from build123d import *

# Parameters (mm, degrees)
CYLINDER003_R     = 1.25
CYLINDER003_DEPTH = 9
CYLINDER002_R     = 1.25
CYLINDER002_DEPTH = 9
BOX008_W          = 5
BOX008_H          = 25
BOX008_DEPTH      = 10
BOX009_W          = 5
BOX009_H          = 5
BOX009_DEPTH      = 2
BOX005_W          = 20
BOX005_H          = 10
BOX005_DEPTH      = 10
CYLINDER_R        = 6.25
CYLINDER_DEPTH    = 5
CYLINDER001_R     = 7.25
CYLINDER001_DEPTH = 5
BOX004_W          = 6.5
BOX004_H          = 7
BOX004_DEPTH      = 10
BOX002_W          = 13.5
BOX002_H          = 10
BOX002_DEPTH      = 12
BOX003_W          = 13
BOX003_H          = 13
BOX003_DEPTH      = 12
BOX_W             = 17
BOX_H             = 23
BOX_DEPTH         = 12
BOX001_W          = 19
BOX001_H          = 25
BOX001_DEPTH      = 10
BOX007_W          = 13
BOX007_H          = 10
BOX007_DEPTH      = 10
BOX006_W          = 15
BOX006_H          = 10
BOX006_DEPTH      = 10
BOX010_W          = 1
BOX010_H          = 10
BOX010_DEPTH      = 1.6


with BuildPart() as cylinder003:
    # Cylinder003 → Cylinder003 (new body)
    with BuildSketch(Plane(origin=(-2, 20, 1), x_dir=(1, 0, 0), z_dir=(0, 0, 1))):
        Circle(CYLINDER003_R)
    extrude(amount=CYLINDER003_DEPTH)


with BuildPart() as cylinder002:
    # Cylinder002 → Cylinder002 (new body)
    with BuildSketch(Plane(origin=(-2, 3, 1), x_dir=(1, 0, 0), z_dir=(0, 0, 1))):
        Circle(CYLINDER002_R)
    extrude(amount=CYLINDER002_DEPTH)


with BuildPart() as cube008:
    # Box008 → Box008 (new body)
    with BuildSketch(Plane(origin=(-5, -1, 0), x_dir=(1, 0, 0), z_dir=(0, 0, 1))):
        with Locations((2.5, 12.5)):
            Rectangle(BOX008_W, BOX008_H)
    extrude(amount=BOX008_DEPTH)


with BuildPart() as cube009:
    # Box009 → Box009 (new body)
    with BuildSketch(Plane(origin=(15, 3, 6), x_dir=(1, 0, 0), z_dir=(0, 0, 1))):
        with Locations((2.5, 2.5)):
            Rectangle(BOX009_W, BOX009_H)
    extrude(amount=BOX009_DEPTH)


with BuildPart() as cube005:
    # Box005 → Box005 (new body)
    with BuildSketch(Plane(origin=(0, 24, 3), x_dir=(1, 0, 0), z_dir=(0, 0, 1))):
        with Locations((10, 5)):
            Rectangle(BOX005_W, BOX005_H)
    extrude(amount=BOX005_DEPTH)


with BuildPart() as cylinder:
    # Cylinder → Cylinder (new body)
    with BuildSketch(Plane(origin=(9.5, 29, 3), x_dir=(1, 0, 0), z_dir=(0, -1, 0))):
        Circle(CYLINDER_R)
    extrude(amount=CYLINDER_DEPTH)


with BuildPart() as cut005:
    # Cylinder001 → Cylinder001 (new body)
    with BuildSketch(Plane(origin=(9.5, 29, 3), x_dir=(1, 0, 0), z_dir=(0, -1, 0))):
        Circle(CYLINDER001_R)
    extrude(amount=CYLINDER001_DEPTH)

    # Cut004: cut Cylinder
    add(cylinder.part, mode=Mode.SUBTRACT)

    # Cut005: cut Cube005
    add(cube005.part, mode=Mode.SUBTRACT)


with BuildPart() as cube004:
    # Box004 → Box004 (new body)
    with BuildSketch(Plane(origin=(15, 10.8, 5), x_dir=(1, 0, 0), z_dir=(0, 0, 1))):
        with Locations((3.25, 3.5)):
            Rectangle(BOX004_W, BOX004_H)
    extrude(amount=BOX004_DEPTH)


with BuildPart() as cube002:
    # Box002 → Box002 (new body)
    with BuildSketch(Plane(origin=(2.75, 15, 1), x_dir=(1, 0, 0), z_dir=(0, 0, 1))):
        with Locations((6.75, 5)):
            Rectangle(BOX002_W, BOX002_H)
    extrude(amount=BOX002_DEPTH)


with BuildPart() as cube003:
    # Box003 → Box003 (new body)
    with BuildSketch(Plane(origin=(3, -1, 2), x_dir=(1, 0, 0), z_dir=(0, 0, 1))):
        with Locations((6.5, 6.5)):
            Rectangle(BOX003_W, BOX003_H)
    extrude(amount=BOX003_DEPTH)


with BuildPart() as cube:
    # Box → Box (new body)
    with BuildSketch(Plane(origin=(1, 0, 1), x_dir=(1, 0, 0), z_dir=(0, 0, 1))):
        with Locations((8.5, 11.5)):
            Rectangle(BOX_W, BOX_H)
    extrude(amount=BOX_DEPTH)


with BuildPart() as fusion:
    # Box001 → Box001 (new body)
    with BuildSketch(Plane(origin=(0, -1, 0), x_dir=(1, 0, 0), z_dir=(0, 0, 1))):
        with Locations((9.5, 12.5)):
            Rectangle(BOX001_W, BOX001_H)
    extrude(amount=BOX001_DEPTH)

    # Cut: cut Cube
    add(cube.part, mode=Mode.SUBTRACT)

    # Cut001: cut Cube003
    add(cube003.part, mode=Mode.SUBTRACT)

    # Cut002: cut Cube002
    add(cube002.part, mode=Mode.SUBTRACT)

    # Cut003: cut Cube004
    add(cube004.part, mode=Mode.SUBTRACT)

    # Fusion: union Cut005
    add(cut005.part)


with BuildPart() as cube007:
    # Box007 → Box007 (new body)
    with BuildSketch(Plane(origin=(3, 14, 1), x_dir=(1, 0, 0), z_dir=(0, 0, 1))):
        with Locations((6.5, 5)):
            Rectangle(BOX007_W, BOX007_H)
    extrude(amount=BOX007_DEPTH)


with BuildPart() as cube006:
    # Box006 → Box006 (new body)
    with BuildSketch(Plane(origin=(2, 13, 1), x_dir=(1, 0, 0), z_dir=(0, 0, 1))):
        with Locations((7.5, 5)):
            Rectangle(BOX006_W, BOX006_H)
    extrude(amount=BOX006_DEPTH)


with BuildPart() as cut010:
    # Cone → Cone (revolve)
    with BuildSketch(Plane(origin=(9.5, 14, 3), x_dir=(1, 0, 0), z_dir=(0, 0, 1))):
        Polygon((0, 0), (4, 0), (7.25, 10), (0, 10), align=None)
    revolve(axis=Axis((9.5, 14, 3), (0, 1, 0)))

    # Cut006: cut Cube006
    add(cube006.part, mode=Mode.SUBTRACT)

    # Cut007: cut Cube007
    add(cube007.part, mode=Mode.SUBTRACT)

    # Fusion001: union Fusion
    add(fusion.part)

    # Cut008: cut Cube009
    add(cube009.part, mode=Mode.SUBTRACT)

    # Fusion002: union Cube008
    add(cube008.part)

    # Cut009: cut Cylinder002
    add(cylinder002.part, mode=Mode.SUBTRACT)

    # Cut010: cut Cylinder003
    add(cylinder003.part, mode=Mode.SUBTRACT)


with BuildPart() as fusion003:
    # Box010 → Box010 (new body)
    with BuildSketch(Plane(origin=(18, 10, 8.4), x_dir=(1, 0, 0), z_dir=(0, 0, 1))):
        with Locations((0.5, 5)):
            Rectangle(BOX010_W, BOX010_H)
    extrude(amount=BOX010_DEPTH)

    # Fusion003: union Cut010
    add(cut010.part)


solid = fusion003.part
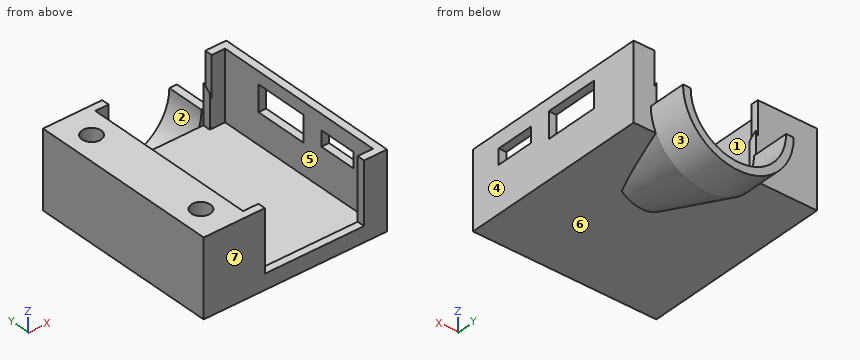
Geometry check sheet. Reference: the model listing, model coordinates, mm. Face numbers are marked on the shaded views. A direction names the side the tool comes from. Round coordinates to 2 decimals unless told otherwise and drop trailing zeros. Loops run counter-clockwise (first coordinate to the right, second up) from the corner with the lowest first, then second, coordinate; pieces in that order, holes last. Notation, with made-up numbers: (27.25, -23) - (59.25, -23) arc R26 ccw to (59.25, 9) - close; hole circle Ø8 at (77, 26.25). An arc over 180 degrees is marked (long way). Answer as CSV lines item,"result".
(1) Set-up check for the marked faces 1, 2, 3 and 4: record each of +Z, -Z, +X, -X, +Y, -Y from which the full face is reachable in a straight line by a thin tool's end or side.
Output values:
face 1,"+Z"
face 2,"+Z, +Y"
face 3,"-Z, +Y"
face 4,"+Z, -Z, +X, +Y, -Y"
(2) Depth check by flat-ended pin: pin 1 Ø1.1 at (x, y) = (16.5, 25.5) entering from +Z; pin 2 Ø2 at (x, y) = (-1.5, 3.5) entering from +Z; pin 3 Ø0.5 at (x, z) = (8.5, -0.5) entering from -Y; pin 4 Ø8 at (x, y) = (5.5, 10) entering from +Z. Enter the tip coordinate at first touch or a pass-through.
Output values:
pin 1,"stops at z = 3"
pin 2,"stops at z = 10"
pin 3,"stops at y = 14"
pin 4,"stops at z = 1"
(3) Cross-section at D-D, the plane x = 9.5. Enter the section's corners in (y, z), and give its area (4 significant figures).
Output values:
outline,"(-1, 0) - (14, 0) - (14, -1) - (24, -4.25) - (29, -4.25) - (29, -3.25) - (24, -3.25) - (24, 1) - (0, 1) - (0, 2) - (-1, 2) - close"
area,"57.25 mm²"
(4) Material ranges on line 1 along Y through (x, z) = (-2, 3.25); line 2 along X through (y, z) = (8.25, 9.25); line 3 along Y through (x, z) = (2.5, 2.75), recorded low to high.
Output values:
line 1,"y = -1 to 1.75, 4.25 to 18.75, 21.25 to 24"
line 2,"x = -5 to 1, 18 to 19"
line 3,"y = -1 to 0, 23 to 29"
(5) Release check for a two-part mould opening along Y. For the marked faces 5, 6 and 7 record: released by +Y, released by -Y, zero draft, split by the parting line, or undercut.
Output values:
face 5,"undercut"
face 6,"zero draft"
face 7,"released by -Y"
(6) Cross-section at C-C, the plane x = -2. Enter the section's corners in (y, z), and give its area (3 significant figures).
Output values:
outline,"(-1, 0) - (24, 0) - (24, 10) - (21.25, 10) - (21.25, 1) - (18.75, 1) - (18.75, 10) - (4.25, 10) - (4.25, 1) - (1.75, 1) - (1.75, 10) - (-1, 10) - close"
area,"205 mm²"
(7) Cross-section at A-A, the plane y = 13. Enter the section's corners in (x, z), and give its area (3 significant figures).
Output values:
outline,"(-5, 0) - (19, 0) - (19, 5) - (18, 5) - (18, 1) - (1, 1) - (1, 10) - (-5, 10) - close; (18, 8.4) - (19, 8.4) - (19, 10) - (18, 10) - close"
area,"83.6 mm²"
(8) Cross-section at B-B, the plane y = 9.5. Enter the section's corners in (x, z), and give its area (3 significant figures).
Output values:
outline,"(-5, 0) - (19, 0) - (19, 10) - (18, 10) - (18, 1) - (1, 1) - (1, 10) - (-5, 10) - close"
area,"87.0 mm²"
